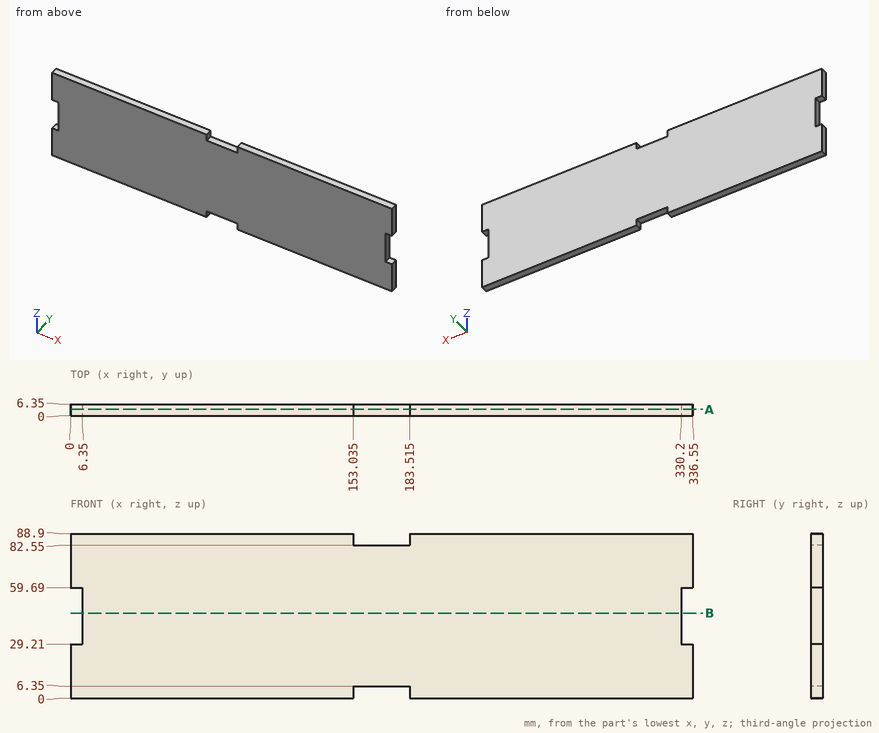
Geometry: see drawing. Coordinates: mm, zero at the bounding-box minimum. Round coordinates to 2 decimals unless told otherwise and drop trailing zeros. Write each loop counter-clockwise with the first axis right and the second up, starting at its lowest first coordinate (ties: lowest second). Pieces come first, ordered by that corner, then holes.
1) Ray query, L1, parallel to Z at x = 161, y = 4.5; L2, parallel to X at y = 0.5, z = 32. Return the intervals inside material, ascending.
2) Cut plane A-A (y = 3.5). Return the cut outline in (x, z) (3 decimals), then the cut area to 3 significant figures.
3) Contact query for flat-ended pins moving along their axis: P1, Ø1, axis at y = 2, z = 53, coming from the -X side; P2, Ø1.9, axis at x = 164, y = 2.5, coming from the +Z side. Output: stop coordinate, or through.
4) Cut plane B-B (z = 46). Return the cut outline in (x, y), then the cut area to 3 significant figures.
Geometry says:
1. L1: z = 6.35 to 82.55
1. L2: x = 6.35 to 330.2
2. outline: (0, 0) - (153.035, 0) - (153.035, 6.35) - (183.515, 6.35) - (183.515, 0) - (336.55, 0) - (336.55, 29.21) - (330.2, 29.21) - (330.2, 59.69) - (336.55, 59.69) - (336.55, 88.9) - (183.515, 88.9) - (183.515, 82.55) - (153.035, 82.55) - (153.035, 88.9) - (0, 88.9) - (0, 59.69) - (6.35, 59.69) - (6.35, 29.21) - (0, 29.21) - close
2. area: 29,100 mm2
3. P1: stops at x = 6.35
3. P2: stops at z = 82.55
4. outline: (6.35, 0) - (330.2, 0) - (330.2, 6.35) - (6.35, 6.35) - close
4. area: 2,060 mm2
